```python
from build123d import *

# Parameters (mm, degrees)
SKETCH1_R           = 19.05
BOSS_EXTRUDE1_DEPTH = 76.2
FILLET2_R           = 2.54
SKETCH2_R           = 1.9939
BOSS_EXTRUDE2_DEPTH = 35.56
SKETCH3_R           = 1.27
CUT_EXTRUDE1_DEPTH  = 35.56


with BuildPart() as part:
    # Sketch1 → Boss-Extrude1 (new body)
    with BuildSketch(Plane.XY):
        with Locations(Location((0, 0, 0), (0, 0, 180))):
            Circle(SKETCH1_R)
    extrude(amount=BOSS_EXTRUDE1_DEPTH)

    # Fillet2
    fillet2_edges = [part.edges().sort_by_distance(p)[0] for p in [
        (19.05, 0, 76.2),
    ]]
    fillet(fillet2_edges, radius=FILLET2_R)

    # Sketch2 → Boss-Extrude2 (add)
    with BuildSketch(Plane.XY.offset(76.2)):
        Circle(SKETCH2_R)
    extrude(amount=BOSS_EXTRUDE2_DEPTH)

    # Sketch3 → Cut-Extrude1 (cut)
    with BuildSketch(Plane.XY.offset(76.2)):
        with Locations((12.7, 0)):
            Circle(SKETCH3_R)
        with Locations((0, -12.7)):
            Circle(SKETCH3_R)
        with Locations((-12.7, 0)):
            Circle(SKETCH3_R)
        with Locations((0, 12.7)):
            Circle(SKETCH3_R)
    extrude(amount=-CUT_EXTRUDE1_DEPTH, mode=Mode.SUBTRACT)


solid = part.part
```
Geometry: final body of the model. Coordinates: model frame, mm. A direction names the side the tool comes from. Round coordinates to 2 decimals unless told otherwise and drop trailing zeros. Loops run counter-clockwise (first coordinate to the right, second up) from the corner with the lowest first, then second, coordinate; pieces in that order, holes last. Notation, with made-up numbers: (30, 32) -> (59, 32) arc R22 cw to (59, 68) -> close; hole circle Ø10 at (12, 28). An arc over 180 degrees is marked (long way). Use one line per item in the form item = value. Start each with the question number.
1) Section A-A on x = 0. Output: boundary loops of the cut face in (y, z), then the cut area to 3 significant figures.
2) First-contact query: P1, Ø4, axis at y = -0.5, z = 83.5, coming from the -X side; P2, Ø10, axis at x = -4.5, z = 46.5, coming from the -Y side; P3, Ø4, axis at y = -10.5, z = 53, coming from the +X side. Flat tips, straight axial feed; report the tip coordinate or a pass-through.
3) Line query: L1, parallel to Y at x = 0, z = 53; L2, parallel to X at y = -12, z = 60; L3, parallel to Y at x = 12.7, z = 57. Output: solid intervals per line, ascending.
4) Section D-D on z = 81.5. Output: boundary loops of the cut face in (x, y), then the cut area to 3 significant figures.
5) Section C-C on z = 27.5. Output: boundary loops of the cut face in (x, y), then the cut area to 3 significant figures.
6) Draft query along X for faces 3 (the flat face through (-13, 0, 40.64)), 4 (the flat face through (0, 0, 0)), 5 (the flat face through (0, 13, 40.64)), 6 (the cylindrical face through (1.9, 0.6, 93.7)). Return one class per face: released by +X, released by -X, zero draft, split by the parting line, or undercut.
7) Section B-B on z = 54.5. Output: boundary loops of the cut face in (x, y).
8) Access query for faces 1 (the cylindrical face through (-13.97, 0.06, 58.67)), 2 (the cylindrical face through (4.13, 18.597, 36.314)). Directions: +Z, -Z, +X, -X, +Y, -Y. A direction counts if a zero-diameter tool reaches every point of the face in a straight line with its end or side. Return the directions, or none.
Response:
q1.outline = (-19.05, 0) -> (19.05, 0) -> (19.05, 73.66) arc R2.54 ccw to (16.51, 76.2) -> (13.97, 76.2) -> (13.97, 40.64) -> (11.43, 40.64) -> (11.43, 76.2) -> (1.99, 76.2) -> (1.99, 111.76) -> (-1.99, 111.76) -> (-1.99, 76.2) -> (-11.43, 76.2) -> (-11.43, 40.64) -> (-13.97, 40.64) -> (-13.97, 76.2) -> (-16.51, 76.2) arc R2.54 ccw to (-19.05, 73.66) -> close
q1.area = 2,860 mm^2
q2.P1 = -1.99
q2.P2 = -19.05
q2.P3 = 17.05
q3.L1 = -19.05 to -13.97, -11.43 to 11.43, 13.97 to 19.05
q3.L2 = -14.8 to -1.06, 1.06 to 14.8
q3.L3 = -14.2 to -1.27, 1.27 to 14.2
q4.outline = circle Ø3.99 at (0, 0)
q4.area = 12.5 mm^2
q5.outline = circle Ø38.1 at (0, 0)
q5.area = 1,140 mm^2
q6.face_3 = undercut
q6.face_4 = zero draft
q6.face_5 = undercut
q6.face_6 = split by the parting line
q7.outline = circle Ø38.1 at (0, 0); hole circle Ø2.54 at (-12.7, 0); hole circle Ø2.54 at (0, -12.7); hole circle Ø2.54 at (0, 12.7); hole circle Ø2.54 at (12.7, 0)
q8.face_1 = +Z
q8.face_2 = +Z, -Z
